Study the drawing (mm; zero at the part's minimum x, y, z) and answer. Coordinates: 2 decimals unless noted, no trailing zeros. Loops run counter-clockwise (first coordinate to the right, second up) from the corner with the lowest first, then second, coordinate; pieces in that order, holes last. Notation, with made-up numbers: (-37, 83.25) - (-3, 83.25) arc R20 cw to (-3, 106.25) - close; hole circle Ø6 at (87.5, 50). An arc over 180 degrees is marked (long way). Put each result on its own line as item: value.
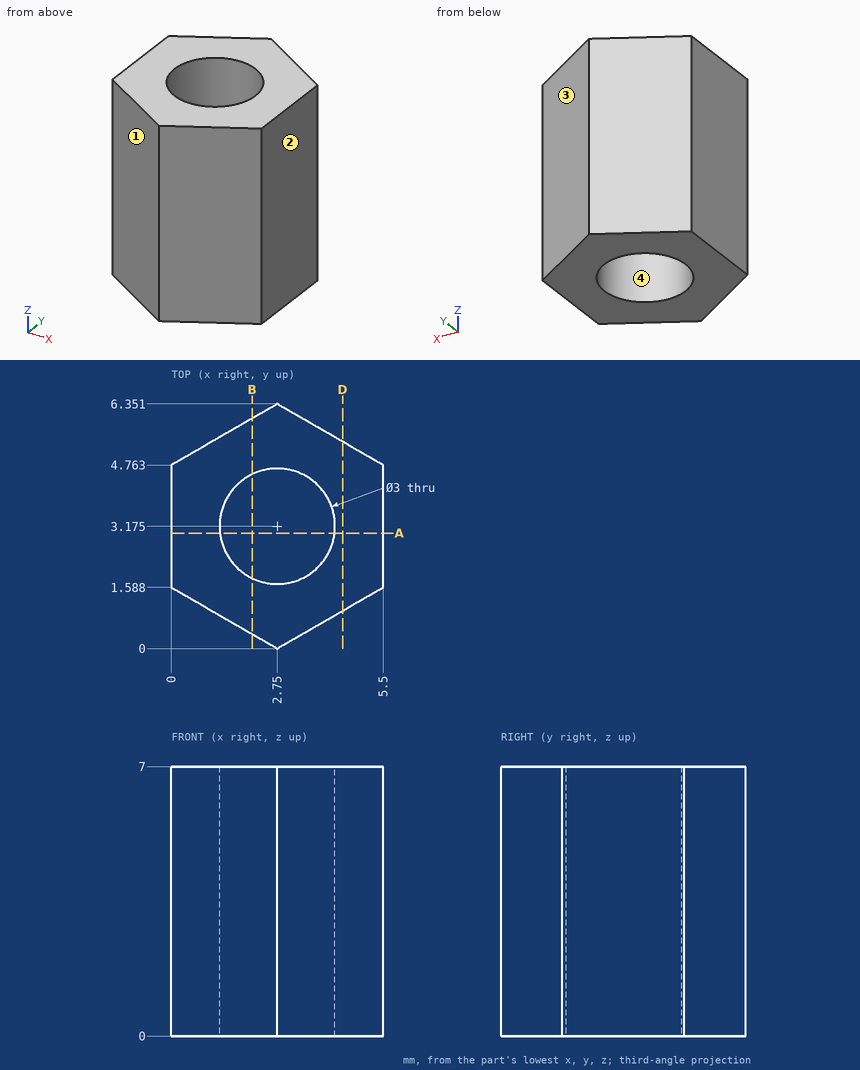
1) The part is cut by section D-D (x = 4.45). Give the vertices of the cut face in (y, z), and give its area (3 significant figures).
Found:
outline: (0.98, 0) - (5.37, 0) - (5.37, 7) - (0.98, 7) - close
area: 30.7 mm^2
2) Each of these flat-tipped pins is pushed along its axis until it touches: pin 1 (1 mm diameter, centred on x = 1, z = 5, fed in from -Y); pin 2 (2 mm diameter, centred on x = 1, z = 2, fed in from +Y); pin 3 (1.5 mm diameter, centred on x = 0.5, z = 2.5, fed in from +Y) (1 decimal). Where does it stop, or does it pass through?
Found:
pin 1: stops at y = 0.72
pin 2: stops at y = 5.92
pin 3: stops at y = 5.5
3) For a pull along Y with two mould halves and no side action, classify the marked faces 1, 2, 3 and 4 as pulls with the +Y half, pulls with the -Y half, needs draft (parallel to the pull), parting line crosses it, or undercut.
Found:
face 1: pulls with the -Y half
face 2: needs draft
face 3: pulls with the +Y half
face 4: undercut
4) Straight lines are drawn through the part: L1, parallel to X at y = 4, z = 5.5 (1 decimal); L2, parallel to Y at x = 1.9, z = 6; L3, parallel to Y at x = 1.5, z = 3.5 (1 decimal). For each, find the intervals that lie inside material, in ascending order. Write a range as [from, to].
Found:
L1: x = [0, 1.5], [4, 5.5]
L2: y = [0.49, 1.94], [4.41, 5.86]
L3: y = [0.7, 2.3], [4, 5.6]
5) The part is cut by section A-A (y = 3). Give the vertices of the cut face in (x, z).
Found:
outline: (0, 0) - (1.26, 0) - (1.26, 7) - (0, 7) - close; (4.24, 0) - (5.5, 0) - (5.5, 7) - (4.24, 7) - close
6) The part is cut by section B-B (x = 2.1). Give the vertices of the cut face in (y, z) (1 decimal).
Found:
outline: (0.4, 0) - (1.8, 0) - (1.8, 7) - (0.4, 7) - close; (4.5, 0) - (6, 0) - (6, 7) - (4.5, 7) - close
